```python
from build123d import *

# Parameters (mm, degrees)
ESBO_O1_W                = 22.8
ESBO_O1_H                = 12
RESSALTO_EXTRUS_O1_DEPTH = 1.6


with BuildPart() as part:
    # Esboço1 → Ressalto-extrusão1 (new body)
    with BuildSketch(Plane.XY):
        with BuildLine():
            Line((-104.371088502, -0.959412185), (-8.45923057, 14.474679896))
            ThreePointArc((-8.45923057, 14.474679896), (-6.836063531, 14.568536185), (-5.227442321, 14.332277754))
            Line((-5.227442321, 14.332277754), (10.244176454, 10.420913457))
            ThreePointArc((10.244176454, 10.420913457), (14.183780118, 8.067281394), (16.181782129, 3.935931872))
            Line((16.181782129, 3.935931872), (17.481460057, -4.140638106))
            ThreePointArc((17.481460057, -4.140638106), (15.894504602, -10.327516352), (10.284415681, -13.380841154))
            Line((10.284415681, -13.380841154), (-9.34255378, -15.108149999))
            ThreePointArc((-9.34255378, -15.108149999), (-9.94330462, -15.138319582), (-10.544624147, -15.123266269))
            Line((-10.544624147, -15.123266269), (-103.02514815, -9.323470085))
            ThreePointArc((-103.02514815, -9.323470085), (-107.880147276, -5.814411311), (-104.371088502, -0.959412185))
        make_face()
        Rectangle(ESBO_O1_W, ESBO_O1_H, mode=Mode.SUBTRACT)
    extrude(amount=RESSALTO_EXTRUS_O1_DEPTH)


solid = part.part
```
Can you work these out from the model? Positions are in its coordinate system, mm. Round coordinates to 2 decimals unless told otherwise and drop trailing zeros. Loops run counter-clockwise (first coordinate to the right, second up) from the corner with the lowest first, then second, coordinate; pieces in that order, holes last. Notation, with made-up numbers: M 74,10.5 L 130,10.5 A14 cw 130,19.5 Z; hole C -19,52.25 d5. An arc over 180 degrees is marked long. Answer in a Markdown table with one row per item.
1. Please list where these lines run through material, in increasing order: line 1 (Y direction, x = 1.5, z = 1.25); line 2 (X direction, y = -3.25, z = 1.35); line 3 (X direction, y = -4.5, z = 0.5). Write a range as from..to.
Established:
| item | result |
|---|---|
| line 1 | -14.15..-6, 6..12.63 |
| line 2 | -107.49..-11.4, 11.4..17.34 |
| line 3 | -107.89..-11.4, 11.4..17.53 |
2. If we section it at B-B, the plane x = 1: Please give me the cut outline in (y, z), plus the area to 3 significant figures.
Established:
| item | result |
|---|---|
| outline | M -14.2,0 L -6,0 L -6,1.6 L -14.2,1.6 Z; M 6,0 L 12.76,0 L 12.76,1.6 L 6,1.6 Z |
| area | 23.9 mm² |
3. If we section it at A-A, the plane y = -2.25: Please give me the cut outline in (x, z).
Established:
| item | result |
|---|---|
| outline | M -106.79,0 L -11.4,0 L -11.4,1.6 L -106.79,1.6 Z; M 11.4,0 L 17.18,0 L 17.18,1.6 L 11.4,1.6 Z |
4. If we section it at D-D, the plane x = -74.5: Please give me the cut outline in (y, z), plus the area to 3 significant figures.
Established:
| item | result |
|---|---|
| outline | M -11.11,0 L 3.85,0 L 3.85,1.6 L -11.11,1.6 Z |
| area | 23.9 mm² |
5. If we section it at C-C, the plane z = 1.25: Please give me the cut outline in (x, y), plus the area to 3 significant figures.
Established:
| item | result |
|---|---|
| outline | M -104.37,-0.96 A4.24 ccw -103.03,-9.32 L -10.54,-15.12 A8 ccw -9.34,-15.11 L 10.28,-13.38 A8 ccw 17.48,-4.14 L 16.18,3.94 A8 ccw 10.24,10.42 L -5.23,14.33 A8 ccw -8.46,14.47 Z; hole M -11.4,-6 L 11.4,-6 L 11.4,6 L -11.4,6 Z |
| area | 2,210 mm² |
6. I'm going to push flat-ended pins straight in: pin 1 Ø0.5 at (y, z) = (-2.5, 0.5) entering from -X; pin 2 Ø0.8 at (x, z) = (-5.5, 0.5) entering from -Y; pin 3 Ø0.5 at (y, z) = (2, 0.5) entering from +X. Where does each tip first touch, or does it pass through?
Established:
| item | result |
|---|---|
| pin 1 | x = -107.19 |
| pin 2 | y = -14.81 |
| pin 3 | x = 16.53 |
